Input: dimensioned drawing with shaded views. Units: mm. Origin: part minimum x, y, z. Round coordinates to 2 decimals unless told otherwise and drop trailing zeros. Loops run counter-clockwise (first coordinate to the right, second up) from the corner with the lowest first, then second, coordinate; pieces in that order, holes last. Notation, with made-up numbers: M 49.5,81 L 59.5,81 A24 cw 59.5,99 Z; hole C 54,23.25 d11. An arc over 180 degrees is marked long. Put each result on its own line as item: value. Start each with the question number.
1) Section B-B on x = 80. Output: boundary loops of the cut face in (y, z) (1 decimal).
2) Draft query along Y for the marked faces 1, 2 and 3. Return one class per face: +Y half, -Y half, draft (parallel to the pull), parting line (faces both ways), or undercut.
3) Section D-D on x = 108.5. Output: boundary loops of the cut face in (y, z), plus the area to 3 significant figures.
4) Section A-A on y = 34. Output: boundary loops of the cut face in (x, z).
5) Line query: probe 1 along X at (y, z) = (64, 3) (1 decimal); probe 2 along X at (y, z) = (86.5, 10.5) (1 decimal); probe 3 along Y at (x, z) = (79.5, 5.25) (1 decimal). Output: solid intervals per line, ascending.
6) Section C-C on z = 1.5. State how many separate pieces and enclosed holes the cut face has.
7) Pin query (flat end, axial travel): pin 1 (5.5 mm diameter, centred on x = 65.86, y = 121.41, fed in from -Z); pin 2 (6 mm diameter, centred on y = 99.5, z = 12, fed in from +X); pin 3 (1.5 mm diameter, centred on x = 115.5, z = 1.5, fed in from -Y); pin 4 (5 mm diameter, centred on y = 81.5, z = 7.5, fed in from +X) (1 decimal). Return the tip coordinate at first contact, or that it passes through.
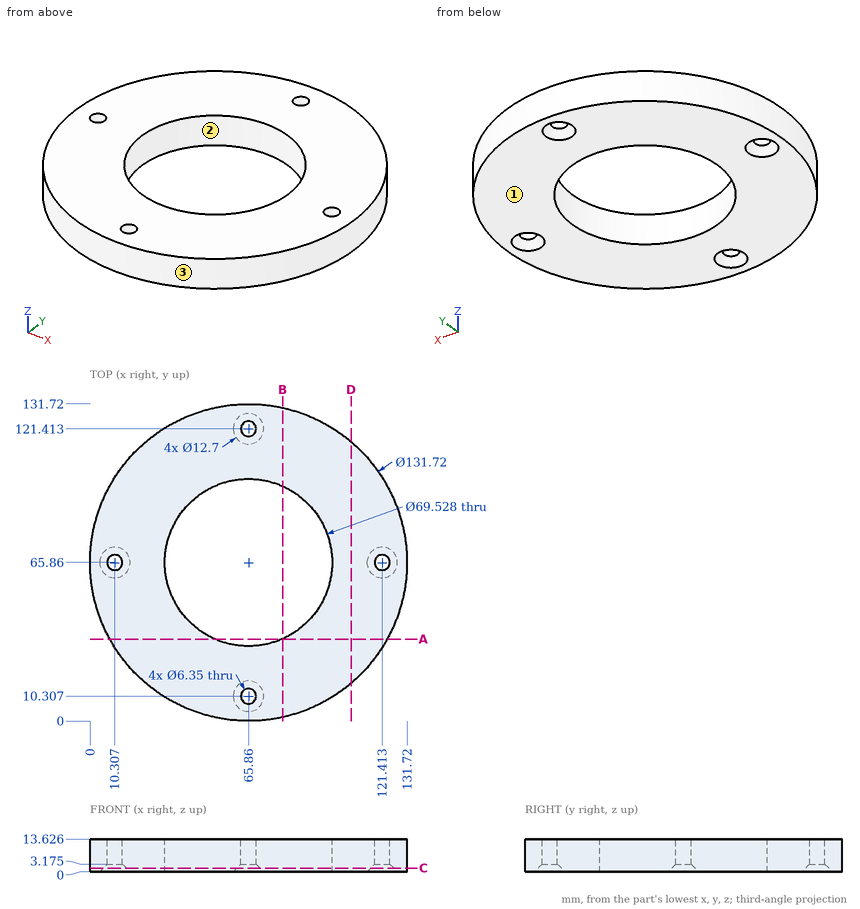
Geometry results:
1. outline: M 1.5,0 L 34.1,0 L 34.1,13.6 L 1.5,13.6 Z; M 97.6,0 L 130.2,0 L 130.2,13.6 L 97.6,13.6 Z
2. face 1: draft
2. face 2: undercut
2. face 3: parting line
3. outline: M 15.67,0 L 116.05,0 L 116.05,13.63 L 15.67,13.63 Z
3. area: 1,370 mm²
4. outline: M 8.22,0 L 51.95,0 L 51.95,13.63 L 8.22,13.63 Z; M 79.77,0 L 123.5,0 L 123.5,13.63 L 79.77,13.63 Z
5. probe 1: x = 0 to 7.5, 13.1 to 31.1, 100.6 to 118.6, 124.2 to 131.7
5. probe 2: x = 3.3 to 37.9, 93.8 to 128.4
5. probe 3: y = 1.4 to 33.9, 97.8 to 130.3
6. separate pieces: 1
6. enclosed holes: 5
7. pin 1: passes through
7. pin 2: stops at x = 124.16
7. pin 3: stops at y = 21.73
7. pin 4: stops at x = 130.4
